Check sheet for the modelled part. Datum: model origin and axes. Units: mm. Face numbers are marked on the shaded views. A direction names the side the tool comes from. Round coordinates to 2 decimals unless told otherwise and drop trailing zeros. Loops run counter-clockwise (first coordinate to the right, second up) from the corner with the lowest first, then second, coordinate; pieces in that order, holes last. Notation, with made-up numbers: (88, 39) - (95, 39) arc R24 cw to (95, 73) - close; hole circle Ø8 at (88, 6.5). An arc over 180 degrees is marked (long way). Return JSON: item names as keys, results as strings.
from build123d import *

# Parameters (mm, degrees)
SKETCH1_R           = 20.9
BOSS_EXTRUDE1_DEPTH = 12
SKETCH2_R           = 1
CUT_EXTRUDE1_DEPTH  = 3
SKETCH3_R           = 1
CUT_EXTRUDE2_DEPTH  = 3
FILLET1_R           = 10
SKETCH4_W           = 15
SKETCH4_H           = 3.988700157
CUT_EXTRUDE3_DEPTH  = 79.126323989
SKETCH8_R           = 1
CUT_EXTRUDE4_DEPTH  = 2


with BuildPart() as part:
    # Sketch1 → Boss-Extrude1 (new body)
    with BuildSketch(Plane(origin=(0, 0, 0), x_dir=(1, 0, 0), z_dir=(0, 1, 0))):
        with BuildLine():
            Line((-41.094820281, 6.777775896), (-45, -16.9))
            Line((-45, -16.9), (-65, -16.9))
            Line((-65, -16.9), (-65, -36.9))
            Line((-65, -36.9), (65, -36.9))
            Line((65, -36.9), (65, -16.9))
            Line((65, -16.9), (45, -16.9))
            Line((45, -16.9), (41.094820281, 6.777775896))
            ThreePointArc((41.094820281, 6.777775896), (0, 41.65), (-41.094820281, 6.777775896))
        make_face()
        with Locations(Location((0, 0, 0), (0, 0, 270))):
            Circle(SKETCH1_R, mode=Mode.SUBTRACT)
    extrude(amount=BOSS_EXTRUDE1_DEPTH)

    # Sketch2 → Cut-Extrude1 (cut)
    with BuildSketch(Plane(origin=(0, 0, 16.9), x_dir=(-1, 0, 0), z_dir=(0, 0, -1))):
        with Locations((-55, 6)):
            Circle(SKETCH2_R)
    extrude(amount=-CUT_EXTRUDE1_DEPTH, mode=Mode.SUBTRACT)

    # Sketch3 → Cut-Extrude2 (cut)
    with BuildSketch(Plane(origin=(0, 0, 16.9), x_dir=(-1, 0, 0), z_dir=(0, 0, -1))):
        with Locations((55, 6)):
            Circle(SKETCH3_R)
    extrude(amount=-CUT_EXTRUDE2_DEPTH, mode=Mode.SUBTRACT)

    # Fillet1
    fillet1_edges = [part.edges().sort_by_distance(p)[0] for p in [
        (-45, 6, 16.9),
        (45, 6, 16.9),
    ]]
    fillet(fillet1_edges, radius=FILLET1_R)

    # Sketch4 → Cut-Extrude3 (cut, through all)
    with BuildSketch(Plane.XZ):
        with Locations((0, -42.963515313)):
            Rectangle(SKETCH4_W, SKETCH4_H)
    extrude(amount=-CUT_EXTRUDE3_DEPTH, mode=Mode.SUBTRACT)

    # Sketch8 → Cut-Extrude4 (cut)
    with BuildSketch(Plane(origin=(0, 0, -40.969165234), x_dir=(-1, 0, 0), z_dir=(0, 0, -1))):
        with Locations((0, 4)):
            Circle(SKETCH8_R)
    extrude(amount=-CUT_EXTRUDE4_DEPTH, mode=Mode.SUBTRACT)


solid = part.part
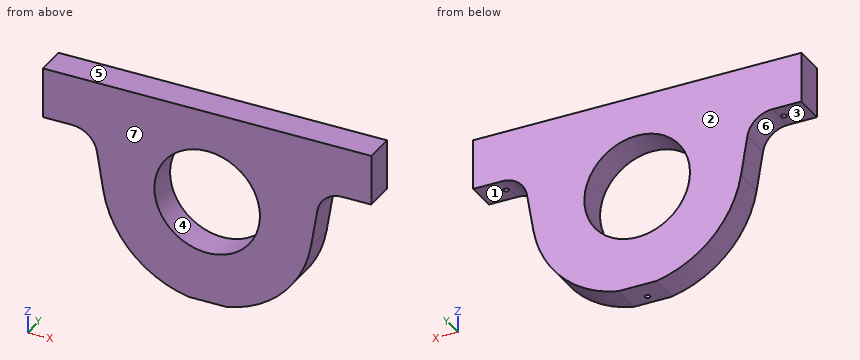
Q1. Sectioned sample at B-B (z = 0). Enter the section's corners in (x, y), plus the area to 3 significant figures.
Answer key:
{"outline": "(-42.21, 0) - (-20.9, 0) - (-20.9, 12) - (-42.21, 12) - close; (20.9, 0) - (42.21, 0) - (42.21, 12) - (20.9, 12) - close", "area": "512 mm²"}
Q2. Sectioned sample at C-C (z = -13). Enter the section's corners in (x, y), plus the area to 3 significant figures.
Answer key:
{"outline": "(-39.57, 0) - (-16.36, 0) - (-16.36, 12) - (-39.57, 12) - close; (16.36, 0) - (39.57, 0) - (39.57, 12) - (16.36, 12) - close", "area": "557 mm²"}
Q3. Depth check by flat-ended pin: P1, Ø3.5, axis at x = 61.5, y = 6, coming from the -Z side; P2, Ø1.8, axis at x = 55, y = 6, coming from the -Z side; P3, Ø5, axis at y = 2, z = -19, coming from the -X side. Enter the tip coordinate at first touch or a pass-through.
Answer key:
{"P1": "stops at z = 16.9", "P2": "stops at z = 19.9", "P3": "stops at x = -38.24"}
Q4. Scan lines: probe 1 along Y at (x, z) = (-55, 17.75); probe 2 along Y at (x, z) = (0, -39); probe 3 along Z at (x, y) = (-58, 9.5). Record each from-to range of solid material in increasing order. Write a range as [from, to].
Answer key:
{"probe 1": "y = [0, 5], [7, 12]", "probe 2": "y = [0, 3], [5, 12]", "probe 3": "z = [16.9, 36.9]"}
Q5. Tool access check on the marked faces 1, 2 and 3. Record the directions out of +Z, -Z, +X, -X, +Y, -Y that give a thin tool (end or side, any length) a straight path to the whole face; none if there is none.
Answer key:
{"face 1": "-Z, +X, +Y, -Y", "face 2": "+Z, -Z, +X, -X, +Y", "face 3": "-Z, -X, +Y, -Y"}
Q6. Draft check along Z on the marked faces 4, 5, 6 and 7. Enter one of: released by +Z, released by -Z, zero draft, split by the parting line, or undercut.
Answer key:
{"face 4": "undercut", "face 5": "released by +Z", "face 6": "released by -Z", "face 7": "zero draft"}
Q7. Sectioned sample at A-A (y = 8.5). Enter the section's corners in (x, z), plus the area to 3 significant figures.
Answer key:
{"outline": "(-65, 16.9) - (-53.49, 16.9) arc R10 cw to (-43.62, 8.53) - (-41.09, -6.78) arc R41.65 ccw to (-7.5, -40.97) - (7.5, -40.97) arc R41.65 ccw to (41.09, -6.78) - (43.62, 8.53) arc R10 cw to (53.49, 16.9) - (65, 16.9) - (65, 36.9) - (-65, 36.9) - close; hole circle Ø41.8 at (0, 0)", "area": "5,450 mm²"}
Q8. Sectioned sample at D-D (x = 39). Enter the section's corners in (y, z).
Answer key:
{"outline": "(0, -14.62) - (12, -14.62) - (12, 36.9) - (0, 36.9) - close"}
